Source: CAD feature listing. Evaluate the final solid. Frame: model axes, mm. A direction names the side the tool comes from. Give positions to 0.01 mm unless a question says otherwise; leave off trailing zeros. Order: outer loops, then holes, each group sorted by start corner. A loop starts at its lowest first (then second) coordinate and runs counter-clockwise, first axis right, second up. Notation, with made-up numbers: (45.5, -16) - (85.5, -16) arc R24 cw to (85.5, -6) - close; hole circle Ø4 at (2, 11). An arc over 180 degrees is marked (long way). Answer as CSV lines item,"result".
```python
from build123d import *

# Parameters (mm, degrees)
F0_R            = 85
F0_R_2          = 1.75
F0_R_3          = 15
F0_R_4          = 5.25
F1_DEPTH        = 2.5
F2_DEPTH        = 2.5
F2_COPIES_COUNT = 4
F3_DEPTH        = 12
F4_DEPTH        = 9
F5_DEPTH        = 3


# Not quite as in the source:
# - a pattern or mirror of a feature is missing from the dataset's text; its kind, count and spacing are read off the source's solid


with BuildPart() as f1:
    # F0 (on Top) → F1 (new body)
    with BuildSketch(Plane.XY):
        Circle(F0_R)
        with Locations((-70.7297637461, -24.9459519848)):
            Circle(F0_R_2, mode=Mode.SUBTRACT)
        Circle(F0_R_3, mode=Mode.SUBTRACT)
        Circle(F0_R_3)
        Circle(F0_R_4, mode=Mode.SUBTRACT)
        Circle(F0_R_4)
        Polygon((-1.2691337593, 2.9107787333), (1.8862414482, 2.554491443), (3.1553752075, -0.3562872903), (1.2691337593, -2.9107787333), (-1.8862414482, -2.554491443), (-3.1553752075, 0.3562872903), align=None, mode=Mode.SUBTRACT)
        Polygon((3.1553752075, -0.3562872903), (1.8862414482, 2.554491443), (-1.2691337593, 2.9107787333), (-3.1553752075, 0.3562872903), (-1.8862414482, -2.554491443), (1.2691337593, -2.9107787333), align=None)
        Circle(F0_R_2, mode=Mode.SUBTRACT)
        with Locations((-70.7297637461, -24.9459519848)):
            Circle(F0_R_2)
    extrude(amount=F1_DEPTH)

    # F0 (on Top) → F2 (cut, through all)
    with BuildSketch(Plane.XY):
        with Locations((-70.7297637461, -24.9459519848)):
            Circle(F0_R_2)
    f2 = extrude(amount=F2_DEPTH, mode=Mode.SUBTRACT)

    # F2_copies: F2 ×4 about axis
    f2_copies_axis = Axis((0, 0, 0), (0, 0, 1))
    for i in range(1, F2_COPIES_COUNT):
        add(f2.rotate(f2_copies_axis, i * 360 / F2_COPIES_COUNT), mode=Mode.SUBTRACT)

    # F0 (on Top) → F3 (join)
    with BuildSketch(Plane.XY):
        Circle(F0_R_4)
        Polygon((-1.2691337593, 2.9107787333), (1.8862414482, 2.554491443), (3.1553752075, -0.3562872903), (1.2691337593, -2.9107787333), (-1.8862414482, -2.554491443), (-3.1553752075, 0.3562872903), align=None, mode=Mode.SUBTRACT)
    extrude(amount=F3_DEPTH)

    # F0 (on Top) → F4 (join)
    with BuildSketch(Plane.XY):
        Polygon((3.1553752075, -0.3562872903), (1.8862414482, 2.554491443), (-1.2691337593, 2.9107787333), (-3.1553752075, 0.3562872903), (-1.8862414482, -2.554491443), (1.2691337593, -2.9107787333), align=None)
        Circle(F0_R_2, mode=Mode.SUBTRACT)
    extrude(amount=F4_DEPTH)

    # F0 (on Top) → F5 (join)
    with BuildSketch(Plane.XY):
        Circle(F0_R_3)
        Circle(F0_R_4, mode=Mode.SUBTRACT)
    extrude(amount=F5_DEPTH)


solid = f1.part
```
(1) Mould query, pull axis Y, two halves, no side actions, for faces 1 (the flat face through (-1.4, -1.3, 9)), 2 (the cylindrical face through (-67.453, -51.721, 1.232)), 3 (the flat face through (-1, -18, 2.5)). Classes: released by +Y, released by -Y, zero draft, split by the parting line, or undercut.
Completed:
face 1,"undercut"
face 2,"split by the parting line"
face 3,"zero draft"
(2) Cut plane D-D (y = -40). Return loops of the section in (x, z).
Completed:
outline,"(-75, 0) - (75, 0) - (75, 2.5) - (-75, 2.5) - close"
(3) Cut plane B-B (z = 7). Return loops of the section in (x, y), then the cut area to 3 significant figures.
Completed:
outline,"circle Ø10.5 at (0, 0); hole circle Ø3.5 at (0, 0)"
area,"77.0 mm²"
(4) Access query for faces 4 (the flat face through (6, 0, 3)), 5 (the flat face through (2.3, -2.3, 12)). Directions: +Z, -Z, +X, -X, +Y, -Y. A direction counts if a zero-diameter tool reaches every point of the face in a straight line with its end or side. Return the directions, or none.
Completed:
face 4,"+Z"
face 5,"+Z, +X, -X, +Y, -Y"
(5) Cut plane C-C (x = 62.5). Return loops of the section in (y, z).
Completed:
outline,"(-57.61, 0) - (57.61, 0) - (57.61, 2.5) - (-57.61, 2.5) - close"
(6) Contact query for flat-ended pins moving along their axis: pin 1 (4 mm diameter, centred on x = 24.95, y = -70.73, fed in from +Z); pin 2 (4 mm diameter, centred on x = -56, z = 2, fed in from +Y); pin 3 (6 mm diameter, centred on x = 21.5, z = 4, fed in from -Y). Output: stop coordinate, or through.
Completed:
pin 1,"z = 2.5"
pin 2,"y = 65.64"
pin 3,"y = -82.87"
(7) Cut plane A-A (y = -12.5). Return loops of the section in (x, z).
Completed:
outline,"(-84.08, 0) - (84.08, 0) - (84.08, 2.5) - (8.29, 2.5) - (8.29, 3) - (-8.29, 3) - (-8.29, 2.5) - (-84.08, 2.5) - close"
(8) Ray query, line 1 (Z direction, x = 15, y = 18.5); line 2 (Z direction, x = -13, y = 1); line 3 (Y direction, x = -69.5, z = 2). Return the intervals inside material, ascending. Write a range as from..to.
Completed:
line 1,"0..2.5"
line 2,"0..3"
line 3,"-48.94..-26.19, -23.7..48.94"
